For this review, take the finished solid that the model builds, in its own axes (mm). Face numbers are marked on the shaded views. A direction names the side the tool comes from. Round coordinates to 2 decimals unless told otherwise and drop trailing zeros. Order: outer loops, then holes, each group sorted by start corner. A loop starts at its lowest first (then second) coordinate and runs counter-clockwise, first axis right, second up. Notation, with made-up numbers: M 8,52 L 60,52 A12 ccw 60,62 Z; hole C 69,-31 d3. An arc over 180 degrees is marked long. Write item = value, one per line. Start each with the question number.
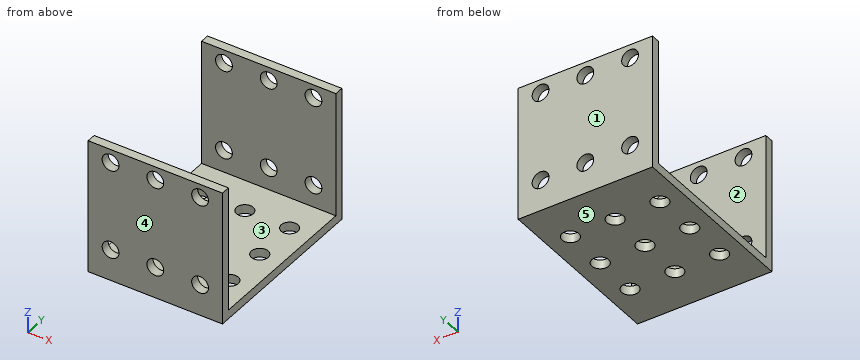
from build123d import *

# Parameters (mm, degrees)
F0_W     = 38.1
F0_H     = 45.72
F0_R     = 2.38125
F1_DEPTH = 2.54
F0_H_2   = 2.54
F2_DEPTH = 38.1
F3_R     = 2.38125
F4_DEPTH = 50.801


with BuildPart() as f1:
    # F0 (on Top) → F1 (new body)
    with BuildSketch(Plane.XY):
        Rectangle(F0_W, F0_H)
        with Locations((-12.7, -12.7)):
            Circle(F0_R, mode=Mode.SUBTRACT)
        with Locations((-12.7, 0)):
            Circle(F0_R, mode=Mode.SUBTRACT)
        with Locations((0, -12.7)):
            Circle(F0_R, mode=Mode.SUBTRACT)
        with Locations((12.7, -12.7)):
            Circle(F0_R, mode=Mode.SUBTRACT)
        Circle(F0_R, mode=Mode.SUBTRACT)
        with Locations((12.7, 0)):
            Circle(F0_R, mode=Mode.SUBTRACT)
        with Locations((-12.7, 12.7)):
            Circle(F0_R, mode=Mode.SUBTRACT)
        with Locations((0, 12.7)):
            Circle(F0_R, mode=Mode.SUBTRACT)
        with Locations((12.7, 12.7)):
            Circle(F0_R, mode=Mode.SUBTRACT)
    extrude(amount=F1_DEPTH)

    # F0 (on Top) → F2 (join)
    with BuildSketch(Plane.XY):
        with Locations((0, 24.13)):
            Rectangle(F0_W, F0_H_2)
        with Locations((0, -24.13)):
            Rectangle(F0_W, F0_H_2)
    extrude(amount=F2_DEPTH)

    # F3 (on face) → F4 (cut, through all)
    with BuildSketch(Plane(origin=(0, 25.4, 0), x_dir=(-1, 0, 0), z_dir=(0, 1, 0))):
        with Locations((-12.7, 34.29)):
            Circle(F3_R)
        with Locations((0, 34.29)):
            Circle(F3_R)
        with Locations((12.7, 34.29)):
            Circle(F3_R)
        with Locations((12.7, 8.89)):
            Circle(F3_R)
        with Locations((0, 8.89)):
            Circle(F3_R)
        with Locations((-12.7, 8.89)):
            Circle(F3_R)
    extrude(amount=-F4_DEPTH, mode=Mode.SUBTRACT)


solid = f1.part
(1) Insertion check: pin 1 (3 mm diameter, centred on x = -5, y = 20, fed in from +Z). The pin has a flat end and moves straight along its axis. Give the tip position at first contact, or say it passes through.
(2) For line 1 along Y through (x, z) = (-12.7, 1.2); line 2 along Y through (x, z) = (0, 17.5); line 3 along X through (y, z) = (-12, 1), list the stretches that pass through material, from the lowest coordinate up.
(3) We need section D-D, the plane x = 5. Write out the cut boundary in (y, z), then the cut area to 3 significant figures.
(4) We need section C-C, the plane z = 8.89. State how many separate pieces and enclosed holes the cut face has, then the cut area to 3 significant figures.
(5) For the marked faces 1 and 2, list the 3-axis set-ups (+Z, -Z, +X, -X, +Y, -Y) from which the entire face can be reached by the end or side of a thin tool; tool diameter is ignored.
(6) Draft analysis for pull direction Y (two halves, no side actions). For the marked faces 3, 4 and 5, state which applies: released by +Y, released by -Y, zero draft, split by the parting line, or undercut.
(7) We need section A-A, the plane y = -12.7. Write out the cut boundary in (x, z).
(8) We need section B-B, the plane z = 3.5. Write out the cut boundary in (x, y), then the cut area to 3 significant figures.
Values:
q1.pin_1 = 2.54
q2.line_1 = -25.4 to -15.08, -10.32 to -2.38, 2.38 to 10.32, 15.08 to 25.4
q2.line_2 = -25.4 to -22.86, 22.86 to 25.4
q2.line_3 = -19.05 to -14.98, -10.42 to -2.28, 2.28 to 10.42, 14.98 to 19.05
q3.outline = M -25.4,0 L 25.4,0 L 25.4,38.1 L 22.86,38.1 L 22.86,2.54 L -22.86,2.54 L -22.86,38.1 L -25.4,38.1 Z
q3.area = 310 mm²
q4.separate_pieces = 8
q4.enclosed_holes = 0
q4.area = 121 mm²
q5.face_1 = +Z, -Z, +X, -X, +Y
q5.face_2 = +Z, +X, -X
q6.face_3 = undercut
q6.face_4 = released by -Y
q6.face_5 = zero draft
q7.outline = M -19.05,0 L -15.08,0 L -15.08,2.54 L -19.05,2.54 Z; M -10.32,0 L -2.38,0 L -2.38,2.54 L -10.32,2.54 Z; M 2.38,0 L 10.32,0 L 10.32,2.54 L 2.38,2.54 Z; M 15.08,0 L 19.05,0 L 19.05,2.54 L 15.08,2.54 Z
q8.outline = M -19.05,-25.4 L 19.05,-25.4 L 19.05,-22.86 L -19.05,-22.86 Z; M -19.05,22.86 L 19.05,22.86 L 19.05,25.4 L -19.05,25.4 Z
q8.area = 194 mm²
